from build123d import *

# Parameters (mm, degrees)
SKETCH1_R           = 46
BOSS_EXTRUDE1_DEPTH = 10
SKETCH2_R           = 12
BOSS_EXTRUDE2_DEPTH = 10
SKETCH3_R           = 3.5
CUT_EXTRUDE1_DEPTH  = 69.058798109
FILLET2_R           = 1
SKETCH4_R           = 33
CUT_EXTRUDE2_DEPTH  = 14
SKETCH9_R           = 7
CUT_EXTRUDE3_DEPTH  = 10
SKETCH10_R          = 2.5
CUT_EXTRUDE4_DEPTH  = 69.058798109
CHAMFER1_SIZE       = 1
SKETCH12_R          = 4
CUT_EXTRUDE7_DEPTH  = 100


with BuildPart() as part:
    # Sketch1 → Boss-Extrude1 (new, symmetric)
    with BuildSketch(Plane.XY):
        Circle(SKETCH1_R)
    extrude(amount=BOSS_EXTRUDE1_DEPTH, both=True)

    # Sketch2 → Boss-Extrude2 (add)
    with BuildSketch(Plane.XY.offset(10)):
        Circle(SKETCH2_R)
    extrude(amount=BOSS_EXTRUDE2_DEPTH)

    # Sketch3 → Cut-Extrude1 (cut, through all)
    with BuildSketch(Plane.XY.offset(10)):
        with Locations((39, 0)):
            Circle(SKETCH3_R)
        with Locations((19.5, -33.774990748)):
            Circle(SKETCH3_R)
        with Locations((-19.5, -33.774990748)):
            Circle(SKETCH3_R)
        with Locations((-39, 0)):
            Circle(SKETCH3_R)
        with Locations((-19.5, 33.774990748)):
            Circle(SKETCH3_R)
        with Locations((19.5, 33.774990748)):
            Circle(SKETCH3_R)
    extrude(amount=-CUT_EXTRUDE1_DEPTH, mode=Mode.SUBTRACT)

    # Fillet2
    fillet2_edges = [part.edges().sort_by_distance(p)[0] for p in [
        (-46, 0, 10),
    ]]
    fillet(fillet2_edges, radius=FILLET2_R)

    # Sketch4 → Cut-Extrude2 (cut)
    with BuildSketch(Plane(origin=(0, 0, -10), x_dir=(-1, 0, 0), z_dir=(0, 0, -1))):
        Circle(SKETCH4_R)
    extrude(amount=-CUT_EXTRUDE2_DEPTH, mode=Mode.SUBTRACT)

    # Sketch9 → Cut-Extrude3 (cut)
    with BuildSketch(Plane.XY.offset(20)):
        Circle(SKETCH9_R)
    extrude(amount=-CUT_EXTRUDE3_DEPTH, mode=Mode.SUBTRACT)

    # Sketch10 → Cut-Extrude4 (cut, through all)
    with BuildSketch(Plane.XY.offset(10)):
        Circle(SKETCH10_R)
    extrude(amount=-CUT_EXTRUDE4_DEPTH, mode=Mode.SUBTRACT)

    # Chamfer1
    chamfer1_edges = [part.edges().sort_by_distance(p)[0] for p in [
        (-7, 0, 20),
    ]]
    chamfer(chamfer1_edges, length=CHAMFER1_SIZE)

    # Sketch12 → Cut-Extrude7 (cut)
    with BuildSketch(Plane(origin=(0, 0, 0), x_dir=(1, 0, 0), z_dir=(0, 1, 0))):
        with Locations(Location((0, 2, 0), (0, 0, 270))):
            Circle(SKETCH12_R)
    extrude(amount=-CUT_EXTRUDE7_DEPTH, mode=Mode.SUBTRACT)


solid = part.part
For this review, take the finished solid that the model builds, in its own axes (mm). A direction names the side the tool comes from. Round coordinates to 2 decimals unless told otherwise and drop trailing zeros. Write each loop counter-clockwise with the first axis right and the second up, starting at its lowest first coordinate (ties: lowest second). Pieces come first, ordered by that corner, then holes. Notation, with made-up numbers: (79.5, 6) - (126.5, 6) arc R5 cw to (126.5, 14) - close; hole circle Ø10 at (-25.75, 78.5). An arc over 180 degrees is marked (long way). Use a Markdown table: item, result.
Q1. We need section B-B (y = 0). State how many separate pieces and enclosed holes the cut face has, plus the area to 3 significant figures.
Derived:
| item | result |
|---|---|
| separate pieces | 4 |
| enclosed holes | 0 |
| area | 705 mm2 |
Q2. We need section A-A (x = 0). Give the boundary of the cut face in (y, z).
Derived:
| item | result |
|---|---|
| outline | (-46, -10) - (-33, -10) - (-33, -6) - (-46, -6) - close; (-46, 2) - (-33, 2) - (-33, 4) - (-2.5, 4) - (-2.5, 10) - (-7, 10) - (-7, 19) - (-8, 20) - (-12, 20) - (-12, 10) - (-45, 10) arc R1 ccw to (-46, 9) - close; (2.5, 4) - (33, 4) - (33, -10) - (46, -10) - (46, 9) arc R1 ccw to (45, 10) - (12, 10) - (12, 20) - (8, 20) - (7, 19) - (7, 10) - (2.5, 10) - close |
Q3. The part is to be moulded in two halves that separate along Z. For faces 4 (the flat face through (9, -9, 10)), 5 (the flat face through (0, -7, 4)), 6 (the cylindrical face through (-3.905, -39.286, -2.867)), say which applies: pulls with the +Z half, pulls with the -Z half, needs draft (parallel to the pull), parting line crosses it, or undercut.
Derived:
| item | result |
|---|---|
| face 4 | pulls with the +Z half |
| face 5 | pulls with the -Z half |
| face 6 | undercut |
Q4. We need section D-D (z = 13.5). Give the boundary of the cut face in (x, y).
Derived:
| item | result |
|---|---|
| outline | circle Ø24 at (0, 0); hole circle Ø14 at (0, 0) |
Q5. Machinability: for faces 1 (the cylindrical face through (35.503, 0.154, 0.14)), 2 (the cylindrical face through (-30.5, -12.6, -3.1)), 3 (the cylindrical face through (6.466, -2.681, 14.563)), which of the approach directions +Z, -Z, +X, -X, +Y, -Y give a long, thin tool a straight path to every point of the face, cutting with its end or side? Answer none if there is none.
Derived:
| item | result |
|---|---|
| face 1 | +Z, -Z |
| face 2 | -Z |
| face 3 | +Z |
Q6. We need section C-C (z = -2). Give the boundary of the cut face in (x, y) (3 decimals), plus the area to 3 significant figures.
Derived:
| item | result |
|---|---|
| outline | (-4, -45.826) - (-4, -32.757) arc R33 cw (long way) to (4, -32.757) - (4, -45.826) arc R46 ccw (long way) to start; hole circle Ø7 at (-39, 0); hole circle Ø7 at (-19.5, -33.775); hole circle Ø7 at (-19.5, 33.775); hole circle Ø7 at (19.5, -33.775); hole circle Ø7 at (19.5, 33.775); hole circle Ø7 at (39, 0) |
| area | 2,890 mm2 |
Q7. Clearance check with flat-ended pins moving along their axes: pin 1 (3 mm diameter, centred on y = -23, z = 2.5, fed in from +X); pin 2 (1 mm diameter, centred on x = -9, y = -10, fed in from -Z); pin 3 (6 mm diameter, centred on x = -16.5, z = 0.5, fed in from -Y). State where each tip first meets the part, or that it passes through.
Derived:
| item | result |
|---|---|
| pin 1 | stops at x = 40.67 |
| pin 2 | stops at z = 4 |
| pin 3 | stops at y = -43.97 |
Q8. Wall thickness on line 1 along X through (y, z) = (-37, 7.5); line 2 along X through (y, z) = (-0.5, 15); line 3 along Y through (x, z) = (-20.5, -3.5): over which ranges is each line inside the solid? List them lowest first.
Derived:
| item | result |
|---|---|
| line 1 | x = -27.33 to -20.86, -18.14 to 18.14, 20.86 to 27.33 |
| line 2 | x = -11.99 to -6.98, 6.98 to 11.99 |
| line 3 | y = -41.18 to -37.13, -30.42 to -25.86, 25.86 to 30.42, 37.13 to 41.18 |
